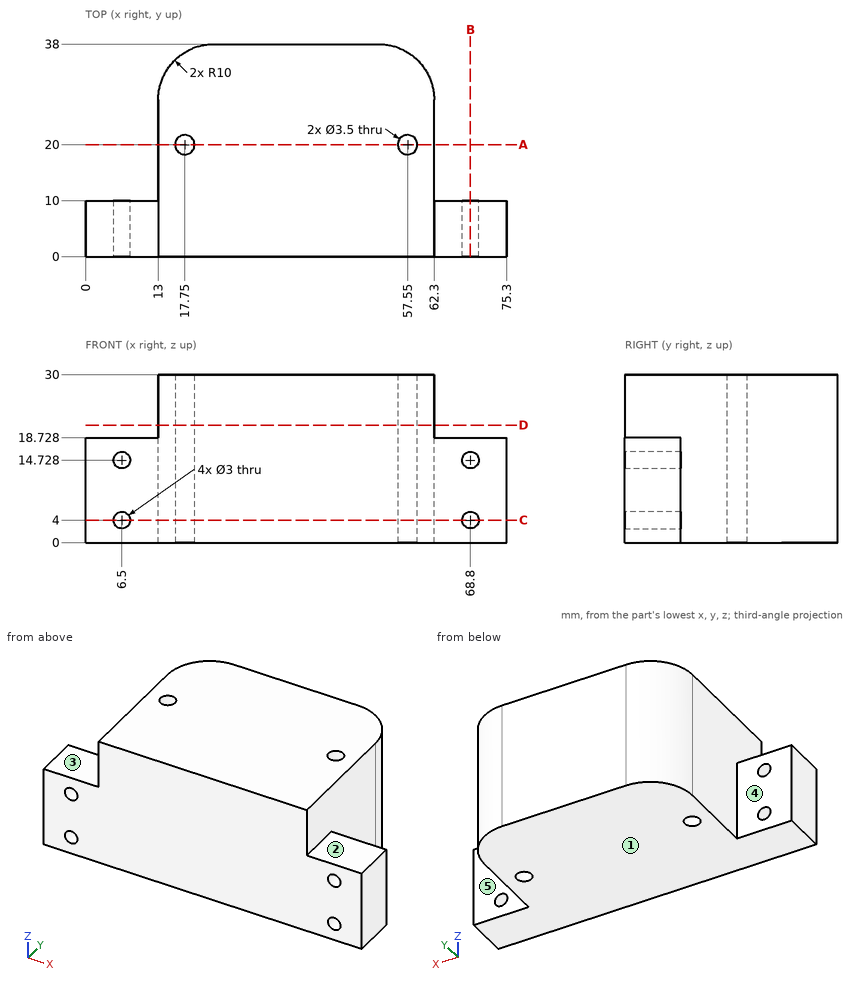
Verification items for this drawing (mm, ordinates from the low corner). A direction names the side the tool comes from. Give positions to 0.01 mm unless a question says otherwise; leave off trailing zeros. Write each loop counter-clockwise with the first axis right and the second up, starting at its lowest first coordinate (ties: lowest second). Pieces come first, ordered by that corner, then holes. Notation, with made-up numbers: (3, -34) -> (14, -34) arc R30 cw to (14, -9) -> close; hole circle Ø6 at (75, 68). An arc over 180 degrees is marked (long way). Use CSV: the item, a comma, the result in double quotes.
(1) Sectioned sample at D-D (z = 21). Record the cut outline in (x, y).
Derived:
outline,"(13, 0) -> (62.3, 0) -> (62.3, 28) arc R10 ccw to (52.3, 38) -> (23, 38) arc R10 ccw to (13, 28) -> close; hole circle Ø3.5 at (17.75, 20); hole circle Ø3.5 at (57.55, 20)"
(2) Sectioned sample at A-A (y = 20). Record the cut outline in (x, z), plus the area to 3 significant figures.
Derived:
outline,"(13, 0) -> (16, 0) -> (16, 30) -> (13, 30) -> close; (19.5, 0) -> (55.8, 0) -> (55.8, 30) -> (19.5, 30) -> close; (59.3, 0) -> (62.3, 0) -> (62.3, 30) -> (59.3, 30) -> close"
area,"1,270 mm^2"
(3) Sectioned sample at B-B (x = 68.8). Record the cut outline in (y, z).
Derived:
outline,"(0, 0) -> (10, 0) -> (10, 2.5) -> (0, 2.5) -> close; (0, 5.5) -> (10, 5.5) -> (10, 13.23) -> (0, 13.23) -> close; (0, 16.23) -> (10, 16.23) -> (10, 18.73) -> (0, 18.73) -> close"
(4) Sectioned sample at C-C (z = 4). Record the cut outline in (x, y), plus the area to 3 significant figures.
Derived:
outline,"(0, 0) -> (5, 0) -> (5, 10) -> (0, 10) -> close; (8, 0) -> (67.3, 0) -> (67.3, 10) -> (62.3, 10) -> (62.3, 28) arc R10 ccw to (52.3, 38) -> (23, 38) arc R10 ccw to (13, 28) -> (13, 10) -> (8, 10) -> close; (70.3, 0) -> (75.3, 0) -> (75.3, 10) -> (70.3, 10) -> close; hole circle Ø3.5 at (17.75, 20); hole circle Ø3.5 at (57.55, 20)"
area,"2,010 mm^2"
(5) Go/stop test with flat-tipped pins: pin 1 (4 mm diameter, centred on x = 6, z = 6, fed in from +Y); pin 2 (8.5 mm diameter, centred on y = 13, z = 22, fed in from +X); pin 3 (5 mm diameter, centred on x = 9, y = 9, fed in from +Z); pin 4 (2.5 mm diameter, centred on x = 68.8, z = 4, fed in from -Y). Record where each tip stops, or that it passes through.
Derived:
pin 1,"stops at y = 10"
pin 2,"stops at x = 62.3"
pin 3,"stops at z = 18.73"
pin 4,"passes through"
(6) Set-up check for the marked faces 1, 2, 3, 4 and 5: record each of +Z, -Z, +X, -X, +Y, -Y from which the full face is reachable in a straight line by a thin tool's end or side.
Derived:
face 1,"-Z, +X, -X, +Y, -Y"
face 2,"+Z, +X, +Y, -Y"
face 3,"+Z, -X, +Y, -Y"
face 4,"+Z, -Z, -X, +Y"
face 5,"+Z, -Z, +X, +Y"
(7) Material ranges on L1, parallel to Z at x = 6.5, y = 6.75; L2, parallel to Y at x = 67.5, z = 8; L3, parallel to X at y = 10, z = 25.75, recorded low to high.
Derived:
L1,"z = 0 to 2.5, 5.5 to 13.23, 16.23 to 18.73"
L2,"y = 0 to 10"
L3,"x = 13 to 62.3"
